Can you work these out from the drawing? Everything is in mm from the part's minimum corner. A direction names the side the tool comes from. Give positions to 0.01 mm unless a question says otherwise; leave off trailing zeros. Write each loop counter-clockwise with the first axis right and the second up, starting at its lowest first coordinate (ties: lowest second). Pieces come first, ordered by that corner, then holes. Notation, with made-up numbers: M 57,-28 L 105,-28 A20 ccw 105,11 Z; hole C 60,-6.75 d9. An arc over 180 degrees is marked long. One line per item, written item: value.
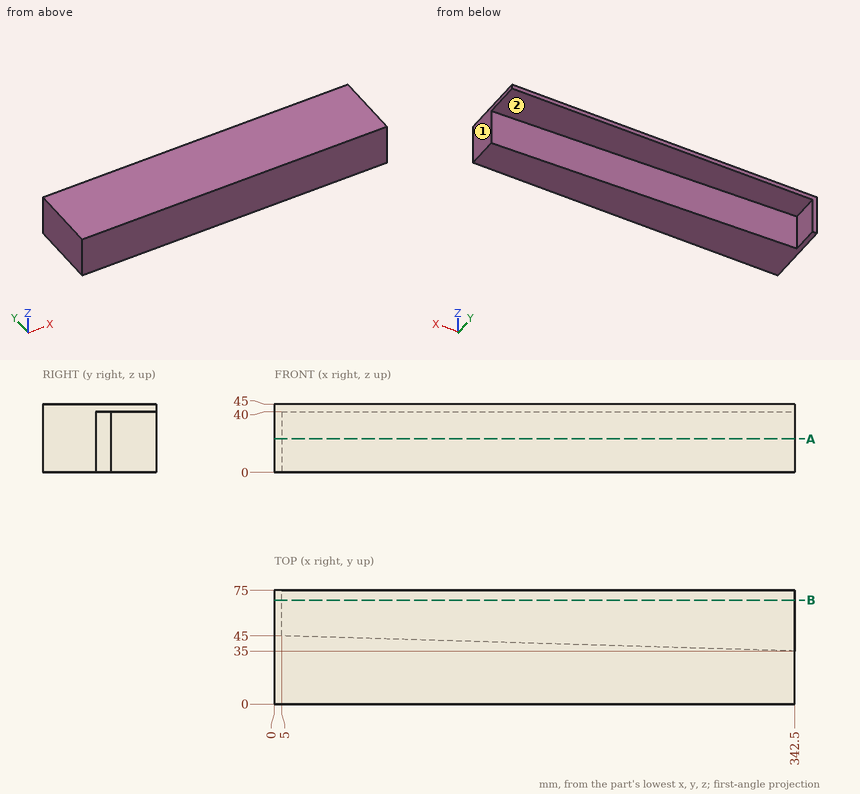
1) On a 3-axis mill with a long thin cutter (end or side, diameter ignored), from which of +Z, -Z, +X, -X, +Y, -Y can I reach the whole of each face in a straight line? I mean the marked faces 1 and 2. Say none if no direction works.
Outcome:
face 1: +Z, -Z, +X, +Y, -Y
face 2: -Z, +X, +Y
2) Please list where these lines run through material, in increasing order: L1, parallel to X at y = 52.5, z = 22; L2, parallel to Z at x = 117, y = 61; L3, parallel to Y at x = 318.5, z = 31.5. Write a range as from..to.
Outcome:
L1: x = 0..5
L2: z = 40..45
L3: y = 0..35.71
3) If we section it at B-B, the plane y = 68.5: Write out the boundary of the cut face in (x, z).
Outcome:
outline: M 0,0 L 5,0 L 5,40 L 342.5,40 L 342.5,45 L 0,45 Z
4) I'm going to push flat-ended pins straight in: pin 1 (1.5 mm diameter, centred on x = 233, y = 49.5, fed in from -Z); pin 2 (12 mm diameter, centred on x = 205.5, z = 31, fed in from +Y); pin 3 (6 mm diameter, centred on x = 251, z = 12, fed in from +Y). Where does each tip first touch, or does it pass through?
Outcome:
pin 1: stops at z = 40
pin 2: stops at y = 39.24
pin 3: stops at y = 37.8
5) If we section it at A-A, the plane z = 22: Write out the boundary of the cut face in (x, y).
Outcome:
outline: M 0,0 L 342.5,0 L 342.5,35 L 5,45 L 5,75 L 0,75 Z
